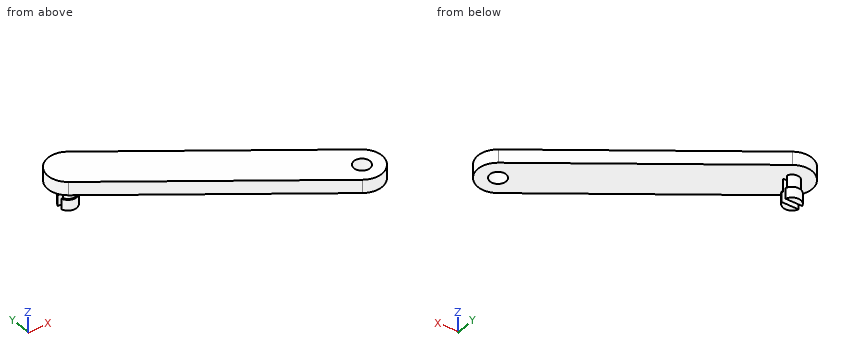
```python
from build123d import *

# Parameters (mm, degrees)
BOSS_EXTRU_1_DEPTH      = 5
ESQUISSE2_R             = 3
ENL_V_MAT_EXTRU_1_DEPTH = 5
ESQUISSE3_R             = 2.75
BOSS_EXTRU_2_DEPTH      = 5
ESQUISSE4_R             = 3.25
BOSS_EXTRU_3_DEPTH      = 4
ESQUISSE5_W             = 10
ESQUISSE5_H             = 2
ENL_V_MAT_EXTRU_2_DEPTH = 9


with BuildPart() as part:
    # Esquisse1 → Boss.-Extru.1 (new body)
    with BuildSketch(Plane.XY):
        with BuildLine():
            Line((15.680221033, -6.131028436), (-56.257179278, 44.554378107))
            ThreePointArc((-56.257179278, 44.554378107), (-58.068428747, 55.00518551), (-47.617621345, 56.816434978))
            Line((-47.617621345, 56.816434978), (24.319778967, 6.131028436))
            ThreePointArc((24.319778967, 6.131028436), (26.131028436, -4.319778967), (15.680221033, -6.131028436))
        make_face()
    extrude(amount=BOSS_EXTRU_1_DEPTH)

    # Esquisse2 → Enlèv. mat.-Extru.1 (cut)
    with BuildSketch(Plane.XY.offset(5)):
        with Locations((20, 0)):
            Circle(ESQUISSE2_R)
    extrude(amount=-ENL_V_MAT_EXTRU_1_DEPTH, mode=Mode.SUBTRACT)

    # Esquisse3 → Boss.-Extru.2 (add)
    with BuildSketch(Plane(origin=(0, 0, 0), x_dir=(-1, 0, 0), z_dir=(0, 0, -1))):
        with Locations(Location((51.937400312, 50.685406543, 0), (0, 0, 180))):
            Circle(ESQUISSE3_R)
    extrude(amount=BOSS_EXTRU_2_DEPTH)

    # Esquisse4 → Boss.-Extru.3 (add)
    with BuildSketch(Plane(origin=(0, 0, -5), x_dir=(-1, 0, 0), z_dir=(0, 0, -1))):
        with Locations((51.937400312, 50.685406543)):
            Circle(ESQUISSE4_R)
    extrude(amount=BOSS_EXTRU_3_DEPTH)

    # Esquisse5 → Enlèv. mat.-Extru.2 (cut)
    with BuildSketch(Plane(origin=(0, 0, -9), x_dir=(-1, 0, 0), z_dir=(0, 0, -1))):
        with Locations((51.937400312, 50.685406543)):
            Rectangle(ESQUISSE5_W, ESQUISSE5_H)
    extrude(amount=-ENL_V_MAT_EXTRU_2_DEPTH, mode=Mode.SUBTRACT)


solid = part.part
```
Work out the finished part from the listing and answer in its coordinate system (mm). Give positions to 0.01 mm unless a question says otherwise; leave off trailing zeros. Order: outer loops, then holes, each group sorted by start corner. A loop starts at its lowest first (then second) coordinate and runs counter-clockwise, first axis right, second up. Notation, with made-up numbers: (3, -13.5) -> (57, -13.5) arc R19 ccw to (57, 14.5) -> close; hole circle Ø2 at (21.25, 31). An arc over 180 degrees is marked (long way). Answer as CSV lines item,"result". Start each with the question number.
(1) Section C-C, the plane y = 0 is taken. Write down the section's boundary in (x, z).
(2) Section D-D, the plane z = -7 is taken. Write down the section's boundary in (x, y), plus the area to 3 significant figures.
(3) Each of these flat-tipped pins is pushed along its axis until it touches: pin 1 Ø5 at (x, z) = (-38, 0) entering from -Y; pin 2 Ø5 at (y, z) = (31.5, 3) entering from +X; pin 3 Ø5.5 at (x, y) = (20, 0) entering from -Z; pin 4 Ø8 at (x, z) = (-28, 1) entering from -Y. Where does it stop, or does it pass through?
(4) Section B-B, the plane x = 20 is taken. Write down the section's boundary in (y, z), plus the area to 3 significant figures.
(5) Consider line 1 along Z through (x, y) = (-29.5, 34.5); line 2 along Y through (x, z) = (-54, -5.25); line 3 along X through (y, z) = (0.5, 3.5). Determine where each line is inside the solid, lowest interval first.
(6) Section A-A, the plane z = 2 is taken. Write down the section's boundary in (x, y).
Entries:
1,outline,"(6.98, 0) -> (17, 0) -> (17, 5) -> (6.98, 5) -> close; (23, 0) -> (27.5, 0) -> (27.5, 5) -> (23, 5) -> close"
2,outline,"(-55.03, 49.69) arc R3.25 ccw to (-48.85, 49.69) -> close; (-55.03, 51.69) -> (-48.85, 51.69) arc R3.25 ccw to start"
2,area,"20.4 mm²"
3,pin 1,"y = 29.93"
3,pin 2,"x = -8.14"
3,pin 3,"through"
3,pin 4,"y = 21.83"
4,outline,"(-7.5, 0) -> (-3, 0) -> (-3, 5) -> (-7.5, 5) -> close; (3, 0) -> (9.17, 0) -> (9.17, 5) -> (3, 5) -> close"
4,area,"53.4 mm²"
5,line 1,"0 to 5"
5,line 2,"48.17 to 49.69, 51.69 to 53.2"
5,line 3,"6.27 to 17.04, 22.96 to 27.48"
6,outline,"(-56.26, 44.55) -> (15.68, -6.13) arc R7.5 ccw to (24.32, 6.13) -> (-47.62, 56.82) arc R7.5 ccw to start; hole circle Ø6 at (20, 0)"
